Geometry check sheet. Reference: the model listing, model coordinates, mm. A direction names the side the tool comes from. Give positions to 0.01 mm unless a question says otherwise; leave off trailing zeros. Write each loop counter-clockwise with the first axis right and the second up, starting at its lowest first coordinate (ties: lowest second). Pieces come first, ordered by that corner, then holes. Notation, with made-up numbers: (-37, 41.25) - (14, 41.25) arc R10 cw to (14, 60.25) - close; hole circle Ø8 at (83.25, -7). An arc over 180 degrees is marked (long way). One line per question, with ' | ' between items. Start each with the question number.
Q1. Thickness scan on L1, parallel to Y at x = -5, z = 1.15; L2, parallel to X at y = 20, z = 4.05; L3, parallel to X at y = 24, z = 2.8. Record the ranges inside material, lowest first. Write a range as [from, to].
Q2. Set-up check for faces 5 (the face through (-20, 16, 2)), 6 (the face through (-17, 5, 2)), 7 (the face through (4, 1, 2)): record each of +Z, -Z, +X, -X, +Y, -Y from which the full face is reachable in a straight line by a thin tool's end or side.
Q3. Gauge pin test, flat ends, axial feed: P1, Ø1.5, axis at y = 1, z = 1.5, coming from the +X side; P2, Ø2.5, axis at x = 9.5, z = 3.5, coming from the -Y side; P3, Ø2.5, axis at y = 3, z = 2, coming from the -X side. Record the tip position at first contact, or that the pin passes through.
Q4. Section check A-A on x = -5. Record the boundary of the cut face in (y, z), and give its area (3 significant figures).
Q5. Section check B-B on y = 23.5. Record the boundary of the cut face in (x, z), and give its area (3 significant figures).
Q6. Section check C-C on z = 1. Record the boundary of the cut face in (x, y), and give its area (3 significant figures).
Q7. Release check for a two-part mould opening along Y. For faces 1 (the face through (1, 32.545, 2)), 2 (the face through (11, 5, 2)), 3 (the face through (-6.11, -3.86, 2.42)), 4 (the face through (-15, 2, 2)) record: +Y half, -Y half, draft (parallel to the pull), parting line (faces both ways), or undercut.
Q8. Section check D-D on y = 5.5. Record the boundary of the cut face in (x, z), and give its area (3 significant figures).
Autodesk Inventor part; units mm, degrees
ref_plane "YZ Plane" through (0, 0, 0) normal (1, 0, 0) x (0, 1, 0)
ref_plane "XZ Plane" through (0, 0, 0) normal (0, 1, 0) x (-1, 0, 0)
ref_plane "XY Plane" through (0, 0, 0) normal (0, 0, 1) x (1, 0, 0)
sketch "Эскиз1" plane through (0, 0, 0) normal (0, 0, 1) x (1, 0, 0)
  line L0 (-20, 5) -> (-20, 27.5449)
  arc A0 (22.2696, 27.5449) -> (17.2696, 32.5449) centre (17.2696, 27.5449) ccw
  line L1 (22.2696, 27.5449) -> (22.2696, 10)
  arc A1 (17.2696, 5) -> (22.2696, 10) centre (17.2696, 10) ccw
  circle A2 centre (-5, -2.85) radius 1.5
  line L2 (-15, 5) -> (-20, 5)
  line L3 (-15, 32.5449) -> (17.2696, 32.5449)
  arc A3 (-15, 32.5449) -> (-20, 27.5449) centre (-15, 27.5449) ccw
  line L4 (17.2696, 5) -> (4, 5)
  arc A4 (0, -6.85) -> (4, -2.85) centre (0, -2.85) ccw
  line L5 (4, -2.85) -> (4, 5)
  line L6 (0, -6.85) -> (-10, -6.85)
  line L7 (-15, -1.85) -> (-15, 5)
  arc A5 (-15, -1.85) -> (-10, -6.85) centre (-10, -1.85) ccw
  circle A6 centre (11.1348, 18.7724) radius 6
  point P0 (22.2696, 32.5449)
  point P1 (0, 32.5449)
  point P2 (22.2696, 5)
  dimension "d14" = 12
  dimension "d15" = 3
extrude "Выдавливание1" add sketch "Эскиз1" along normal blind 4.9
properties part number "Верт. держатели"
Working result:
1) L1: y = [-6.85, -4.35], [-1.35, 32.54] | L2: x = [-20, 5.26], [17.01, 22.27] | L3: x = [-20, 8.19], [14.08, 22.27]
2) face 5: +Z, -Z, -X, +Y, -Y | face 6: +Z, -Z, -X, -Y | face 7: +Z, -Z, +X, -Y
3) P1: stops at x = 4 | P2: stops at y = 5 | P3: stops at x = -15
4) outline: (-6.85, 0) - (-4.35, 0) - (-4.35, 4.9) - (-6.85, 4.9) - close; (-1.35, 0) - (32.54, 0) - (32.54, 4.9) - (-1.35, 4.9) - close | area: 178 mm2
5) outline: (-20, 0) - (7.44, 0) - (7.44, 4.9) - (-20, 4.9) - close; (14.83, 0) - (22.27, 0) - (22.27, 4.9) - (14.83, 4.9) - close | area: 171 mm2
6) outline: (-20, 5) - (-15, 5) - (-15, -1.85) arc R5 ccw to (-10, -6.85) - (0, -6.85) arc R4 ccw to (4, -2.85) - (4, 5) - (17.27, 5) arc R5 ccw to (22.27, 10) - (22.27, 27.54) arc R5 ccw to (17.27, 32.54) - (-15, 32.54) arc R5 ccw to (-20, 27.54) - close; hole circle Ø3 at (-5, -2.85); hole circle Ø12 at (11.13, 18.77) | area: 1,240 mm2
7) face 1: +Y half | face 2: -Y half | face 3: undercut | face 4: draft
8) outline: (-20, 0) - (19.45, 0) - (19.45, 4.9) - (-20, 4.9) - close | area: 193 mm2
